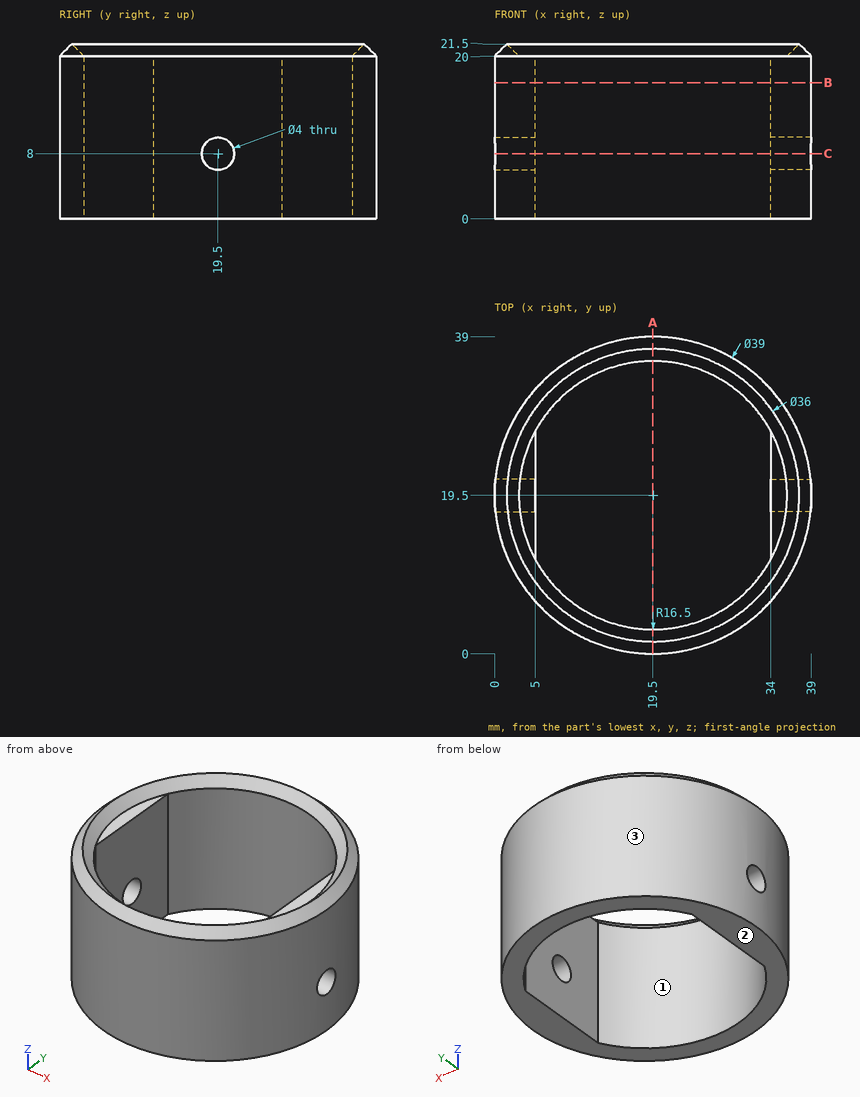
Check sheet for the drawn part. Datum: minimum x, y, z corner. Units: mm. Round coordinates to 2 decimals unless told otherwise and drop trailing zeros. Loops run counter-clockwise (first coordinate to the right, second up) from the corner with the lowest first, then second, coordinate; pieces in that order, holes last.
Item 1: Cross-section at C-C on z = 8. Record the boundary of the cut face in (x, y), then the cut area to 3 significant figures.
Item 2: Cross-section at A-A on x = 19.5. Record the boundary of the cut face in (y, z), then the cut area to 4 significant figures.
Item 3: Cross-section at B-B on z = 16.75. Record the boundary of the cut face in (x, y), then the cut area to 3 significant figures.
Item 4: Gauge pin test, flat ends, axial feed: pin 1 (4 mm diameter, centred on x = 25.5, z = 6, fed in from +Y); pin 2 (6.5 mm diameter, centred on y = 19.5, z = 8, fed in from +X); pin 3 (0.6 mm diameter, centred on x = 4.5, y = 19, fed in from +Z); pin 4 (2 mm diameter, centred on x = 15, z = 14, fed in from +Y). Record the tip position at first contact, or that the pin passes through.
Item 5: Mould release check, pull along Y, two halves, no side actions. Record for the marked faces 1, 2 and 3: pulls with the +Y half, pulls with the -Y half, needs draft (parallel to the pull), parting line crosses it, or undercut.
Item 6: Thickness scan on line 1 (Y direction, x = 20, z = 15.25); line 2 (X direction, y = 5, z = 18); line 3 (Z direction, x = 3.25, y = 19.5). Record the ranges inside material, lowest first.
Answer sheet:
1. outline: (0.1, 17.5) arc R19.5 ccw to (38.9, 17.5) - (34, 17.5) - (34, 11.63) arc R16.5 cw to (5, 11.63) - (5, 17.5) - close; (0.1, 21.5) - (5, 21.5) - (5, 27.37) arc R16.5 cw to (34, 27.37) - (34, 21.5) - (38.9, 21.5) arc R19.5 ccw to start
1. area: 342 mm2
2. outline: (0, 0) - (3, 0) - (3, 20) - (1.5, 21.5) - (0, 20) - close; (36, 0) - (39, 0) - (39, 20) - (37.5, 21.5) - (36, 20) - close
2. area: 124.5 mm2
3. outline: circle Ø39 at (19.5, 19.5); hole (5, 11.63) arc R16.5 ccw to (34, 11.63) - (34, 27.37) arc R16.5 ccw to (5, 27.37) - close
3. area: 382 mm2
4. pin 1: stops at y = 38.59
4. pin 2: stops at x = 39
4. pin 3: stops at z = 20
4. pin 4: stops at y = 38.68
5. face 1: undercut
5. face 2: needs draft
5. face 3: parting line crosses it
6. line 1: y = 0.01 to 3.01, 35.99 to 38.99
6. line 2: x = 6.46 to 11.63, 27.37 to 32.54
6. line 3: z = 0 to 6, 10 to 20
